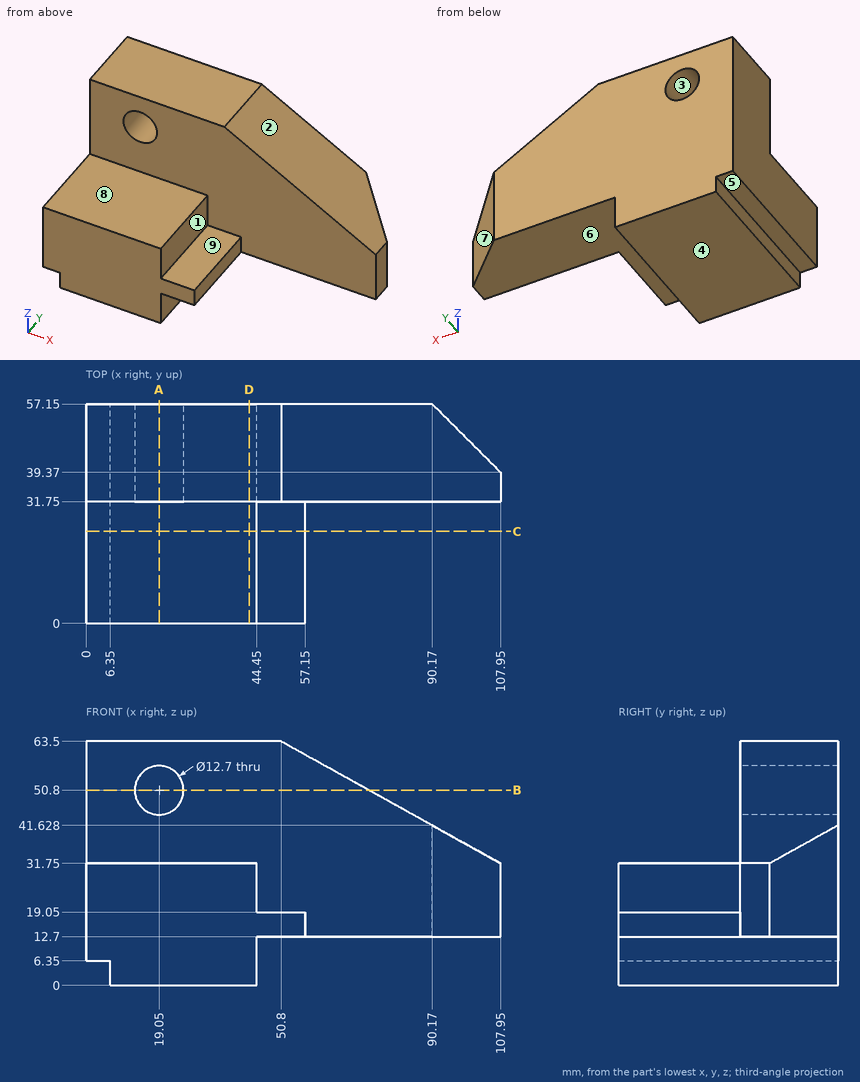
Geometry check sheet. Reference: drawing and pictorial views, mm from the part's lowest x, y, z. A direction names the side the tool comes from. Give positions to 0.01 mm unless a question says otherwise; leave off trailing zeros. Loops run counter-clockwise (first coordinate to the right, second up) from the corner with the lowest first, then second, coordinate; pieces in that order, holes last. Notation, with made-up numbers: (60, 52) - (116, 52) arc R34 ccw to (116, 86) - close; hole circle Ø2 at (9, -15). An arc over 180 degrees is marked (long way). One line per question, with ' | ' between items. Start each with the question number.
1. Cross-section at A-A, the plane x = 19.05. Enter the section's corners in (y, z).
2. Cross-section at B-B, the plane z = 50.8. Enter the section's corners in (x, y).
3. Gauge pin test, flat ends, axial feed: pin 1 Ø7 at (y, z) = (30.5, 2) entering from -X; pin 2 Ø1.9 at (x, y) = (2, 22.5) entering from -Z; pin 3 Ø6.5 at (x, y) = (50.5, 17) entering from +Z. Record the tip position at first contact, or that the pin passes through.
4. Set-up check for the marked faces 5, 6, 7, 8 and 9: record each of +Z, -Z, +X, -X, +Y, -Y from which the full face is reachable in a straight line by a thin tool's end or side.
5. Cross-section at D-D, the plane x = 42.5. Enter the section's corners in (y, z).
6. Draft check along Z on the marked faces 1, 2, 3 and 4. Enter one of: released by +Z, released by -Z, zero draft, split by the parting line, or undercut.
7. Material ranges on line 1 along Z through (x, y) = (19.05, 47.75); line 2 along Y through (x, z) = (10, 36); line 3 along Z through (x, y) = (5, 21), recorded low to high. Write a range as [from, to].
8. Cross-section at C-C, the plane y = 24. Enter the section's corners in (x, z), plus the area to 3 significant figures.
Check result:
1) outline: (0, 0) - (57.15, 0) - (57.15, 44.45) - (31.75, 44.45) - (31.75, 31.75) - (0, 31.75) - close; (31.75, 57.15) - (57.15, 57.15) - (57.15, 63.5) - (31.75, 63.5) - close
2) outline: (0, 31.75) - (12.7, 31.75) - (12.7, 57.15) - (0, 57.15) - close; (25.4, 31.75) - (73.66, 31.75) - (73.66, 57.15) - (25.4, 57.15) - close
3) pin 1: stops at x = 6.35 | pin 2: stops at z = 6.35 | pin 3: stops at z = 19.05
4) face 5: -Z, -X, +Y, -Y | face 6: -Z, +X, +Y, -Y | face 7: +Z, -Z, +X, +Y | face 8: +Z, +X, -X, -Y | face 9: +Z, +X, -Y
5) outline: (0, 0) - (57.15, 0) - (57.15, 63.5) - (31.75, 63.5) - (31.75, 31.75) - (0, 31.75) - close
6) face 1: zero draft | face 2: released by +Z | face 3: undercut | face 4: released by -Z
7) line 1: z = [0, 44.45], [57.15, 63.5] | line 2: y = [31.75, 57.15] | line 3: z = [6.35, 31.75]
8) outline: (0, 6.35) - (6.35, 6.35) - (6.35, 0) - (44.45, 0) - (44.45, 12.7) - (57.15, 12.7) - (57.15, 19.05) - (44.45, 19.05) - (44.45, 31.75) - (0, 31.75) - close | area: 1,450 mm2
